Work out the finished part from the listing and answer in its coordinate system (mm). Give positions to 0.01 mm unless a question says otherwise; leave off trailing zeros. Loops run counter-clockwise (first coordinate to the right, second up) from the corner with the lowest first, then second, coordinate; pieces in that order, holes last. Notation, with made-up numbers: M 18.25,65.25 L 23.25,65.25 A14 cw 23.25,83.25 Z; hole C 75,47 d11. An arc over 180 degrees is marked long. Write item = value, one per line. Start each with the question number.
1. Section D-D on y = -11 is taken. Determine the outline of the cut face in (x, z).
2. Section C-C on y = 0 is taken. Determine the outline of the cut face in (x, z), plus the area to 3 significant figures.
3. Consider L1, parallel to Y at x = 0, z = 17; L2, parallel to Y at x = 18, z = 36.5; L3, parallel to Y at x = 33, z = 12. Determine where each line is inside the solid, lowest interval first. Write a range as [from, to].
4. Section A-A on z = 3 is taken. Determine the outline of the cut face in (x, y).
5. Flat-ended cylindrical pins translate along their axes: pin 1 Ø21 at (x, z) = (2, 28) entering from -Y; pin 2 Ø1 at (y, z) = (-12.5, 24.5) entering from +X; pin 3 Ø5 at (y, z) = (-43.5, 29) entering from +X. Find the tip coordinate at first contact, or state that the pin passes through.
6. Section B-B on x = 0 is taken. Determine the outline of the cut face in (y, z), plus the area to 3 significant figures.
```python
from build123d import *

# Parameters (mm, degrees)
SKETCH1_R           = 50.8
SKETCH1_R_2         = 2.06375
BOSS_EXTRUDE1_DEPTH = 41.656
SKETCH2_W           = 75.184
SKETCH2_H           = 3.302
SKETCH2_W_2         = 95.173769496
SKETCH2_H_2         = 48.323916003
CUT_EXTRUDE6_DEPTH  = 76.2
FILLET1_R           = 2.54
FILLET3_R           = 25.4


with BuildPart() as part:
    # Sketch1 → Boss-Extrude1 (new body)
    with BuildSketch(Plane.XY):
        Circle(SKETCH1_R)
        Circle(SKETCH1_R_2, mode=Mode.SUBTRACT)
    extrude(amount=BOSS_EXTRUDE1_DEPTH)

    # Sketch2 → Cut-Extrude6 (cut)
    with BuildSketch(Plane(origin=(0, 0, 0), x_dir=(-1, 0, 0), z_dir=(0, 0, -1))):
        with Locations((-12.232804706, -11.557)):
            Rectangle(SKETCH2_W, SKETCH2_H)
        with Locations((0, 41.941958002)):
            Rectangle(SKETCH2_W_2, SKETCH2_H_2)
    extrude(amount=-CUT_EXTRUDE6_DEPTH, mode=Mode.SUBTRACT)

    # Fillet1
    fillet1_edges = [part.edges().sort_by_distance(p)[0] for p in [
        (49.052917711, -13.208, 20.828),
        (49.824804706, -9.906, 20.828),
    ]]
    fillet(fillet1_edges, radius=FILLET1_R)

    # Fillet3
    # the kernel refuses this fillet: 25.4 mm, written as the material it takes off along each edge
    with BuildSketch(Plane(origin=(47.586884748, 17.78, -64.168841163), x_dir=(0.1019926357447357, -0.9947851538165624, 0), z_dir=(0, 0, 1))) as fillet3_piece_1:
        with BuildLine():
            CenterArc((22.943972331, -25.253558134), FILLET3_R, 83.844514986, 90.301558127)
            Line((-2.323570576, -22.662945186), (0, 0))
            ThreePointArc((0, 0), (12.833768233, 1.647844473), (25.667536465, 0))
        make_face()
    extrude(amount=169.993682325, mode=Mode.SUBTRACT)
    with BuildSketch(Plane(origin=(-47.586884748, 17.78, -82.578860977), x_dir=(1, 0, 0), z_dir=(0, 0, 1))) as fillet3_piece_2:
        with BuildLine():
            CenterArc((23.356829032, -25.4), FILLET3_R, 90, 107.457603124)
            ThreePointArc((-0.873226684, -33.02), (-3.195360858, -16.437043854), (0, 0))
            Line((0, 0), (23.356829032, 0))
        make_face()
    extrude(amount=206.813721954, mode=Mode.SUBTRACT)


solid = part.part
```
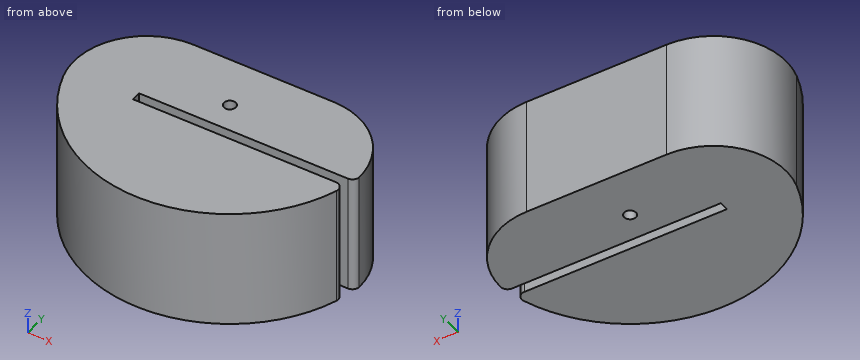
Verdict:
q1.outline = M -49.4,0 L -25.36,0 L -25.36,41.66 L -49.4,41.66 Z
q2.outline = M -48.46,0 L -2.06,0 L -2.06,41.66 L -48.46,41.66 Z; M 2.06,0 L 49.04,0 L 49.04,41.66 L 2.06,41.66 Z
q2.area = 3,890 mm2
q3.L1 = [-50.8, -13.21], [-9.91, -2.06], [2.06, 17.78]
q3.L2 = [-47.5, -13.21], [-9.91, 17.78]
q3.L3 = [-38.62, -13.21], [-9.91, 16.42]
q4.outline = M -48.46,-15.24 A50.8 ccw 48.02,-16.58 A2.54 ccw 45.62,-13.21 L -25.36,-13.21 L -25.36,-9.91 L 47.69,-9.91 A2.54 ccw 50.2,-7.75 A25.4 ccw 24.81,17.78 L -24.23,17.78 A25.4 ccw Z; hole C 0,0 d4.13
q5.pin_1 = -50.8
q5.pin_2 = -25.36
q5.pin_3 = 29.99
q6.outline = M -50.8,0 L -13.21,0 L -13.21,41.66 L -50.8,41.66 Z; M -9.91,0 L -2.06,0 L -2.06,41.66 L -9.91,41.66 Z; M 2.06,0 L 17.78,0 L 17.78,41.66 L 2.06,41.66 Z
q6.area = 2,550 mm2
